Check sheet for the drawn part. Datum: minimum x, y, z corner. Units: mm. Round coordinates to 2 decimals unless told otherwise and drop trailing zeros. Order: outer loops, then holes, each group sorted by start corner. A loop starts at its lowest first (then second) coordinate and runs counter-clockwise, first axis right, second up.
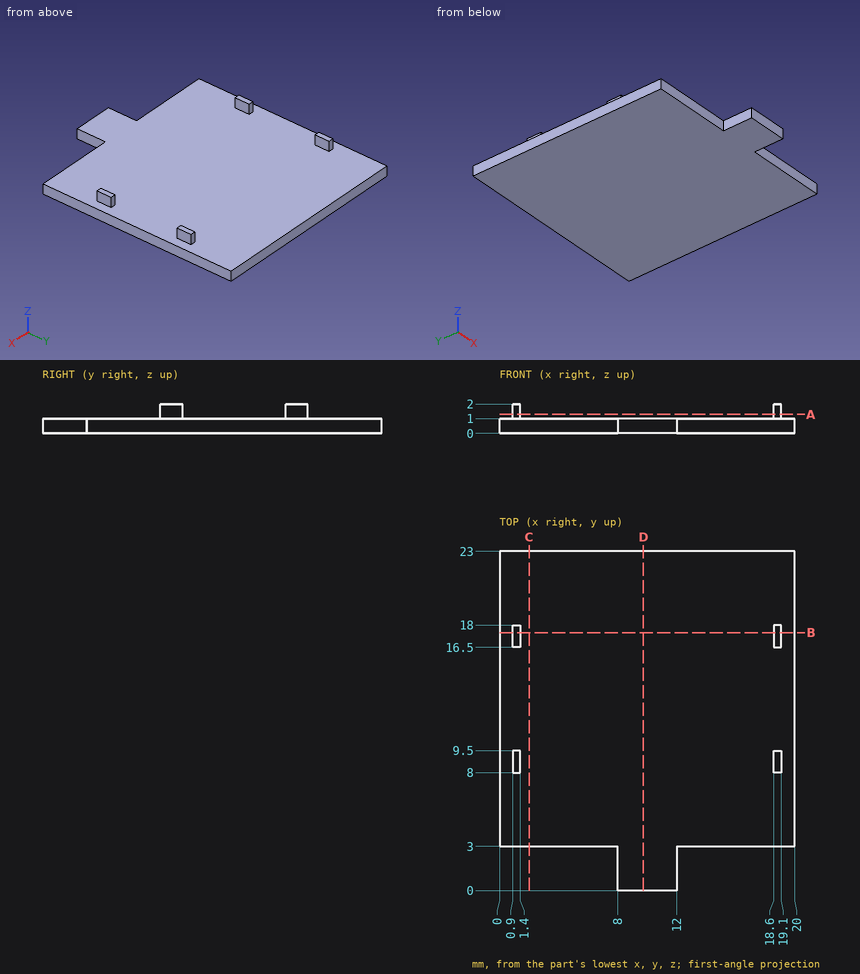
(1) Sectioned sample at D-D, the plane x = 9.75. Record the cut outline in (y, z).
Returned:
outline: (0, 0) - (23, 0) - (23, 1) - (0, 1) - close
(2) Sectioned sample at C-C, the plane x = 2. Record the cut outline in (y, z), and give its area (3 significant figures).
Returned:
outline: (3, 0) - (23, 0) - (23, 1) - (3, 1) - close
area: 20.0 mm2
(3) Material ranges on line 1 (X direction, y = 16.75, z = 1.15); line 2 (Y direction, x = 6, z = 0.9); line 3 (Z direction, x = 2.5, y = 3.5), recorded low to high.
Returned:
line 1: x = 0.9 to 1.4, 18.6 to 19.1
line 2: y = 3 to 23
line 3: z = 0 to 1
(4) Sectioned sample at A-A, the plane z = 1.3. Record the cut outline in (x, y).
Returned:
outline: (0.9, 8) - (1.4, 8) - (1.4, 9.5) - (0.9, 9.5) - close; (0.9, 16.5) - (1.4, 16.5) - (1.4, 18) - (0.9, 18) - close; (18.6, 8) - (19.1, 8) - (19.1, 9.5) - (18.6, 9.5) - close; (18.6, 16.5) - (19.1, 16.5) - (19.1, 18) - (18.6, 18) - close
(5) Depth check by flat-ended pin: P1, Ø1.1, axis at y = 1, z = 0.5, coming from the -X side; P2, Ø6, axis at x = 7, y = 2.5, coming from the +Z side; P3, Ø0.5, axis at y = 8.5, z = 1.5, coming from the -X side. Enter the tip coordinate at first touch or a pass-through.
Returned:
P1: stops at x = 8
P2: stops at z = 1
P3: stops at x = 0.9
(6) Sectioned sample at B-B, the plane y = 17.5. Record the cut outline in (x, z).
Returned:
outline: (0, 0) - (20, 0) - (20, 1) - (19.1, 1) - (19.1, 2) - (18.6, 2) - (18.6, 1) - (1.4, 1) - (1.4, 2) - (0.9, 2) - (0.9, 1) - (0, 1) - close
